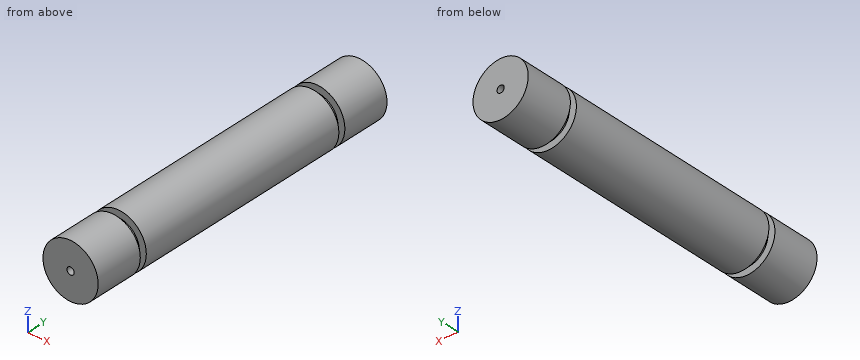
Autodesk Inventor part; units mm, degrees
ref_plane "YZ Plane" through (0, 0, 0) normal (1, 0, 0) x (0, 1, 0)
ref_plane "XZ Plane" through (0, 0, 0) normal (0, 1, 0) x (-1, 0, 0)
ref_plane "XY Plane" through (0, 0, 0) normal (0, 0, 1) x (1, 0, 0)
sketch "Sketch1" plane through (0, 0, 0) normal (0, 0, 1) x (1, 0, 0)
  line L0 (0, 0) -> (25.4, 0)
  line L1 (25.4, 304.8) -> (0, 304.8)
  line L2 (0, 304.8) -> (0, 0)
  line L3 (25.4, 44.45) -> (19.05, 44.45)
  line L4 (19.05, 44.45) -> (19.05, 50.8)
  line L5 (19.05, 50.8) -> (25.4, 50.8)
  line L6 (25.4, 254) -> (19.05, 254)
  line L7 (19.05, 254) -> (19.05, 260.35)
  line L8 (19.05, 260.35) -> (25.4, 260.35)
  line L9 (25.4, 260.35) -> (25.4, 304.8)
  line L10 (25.4, 0) -> (25.4, 44.45)
  line L11 (25.4, 50.8) -> (25.4, 254)
  point P0 (12.7, 152.4)
  point P1 (12.7, 0)
  dimension "d3" = 6.35
  dimension "d4" = 6.35
  dimension "d5" = 6.35
  dimension "d7" = 6.35
  dimension "d8" = 25.4
  dimension "d9" = 25.4
  dimension "d10" = 25.4
  dimension "d11" = 304.8
  dimension "d12" = 152.4
  dimension "d13" = 101.6
  dimension "d14" = 101.6
revolve "Revolution1" add sketch "Sketch1" angle 360 about axis through (0, 304.8, 0) along (0, -1, 0)
sketch "Sketch2" plane through (0, 304.8, 0) normal (0, 1, 0) x (1, 0, 0)
  point P0 (0, 0)
  point P1 (0, 0)
hole "Hole1" at (0, 304.8, 0) direction (0, -1, 0) diameter 6.604 end through all
properties part number "Roller" material "PVC-Piping"
Design review of the part built by this model. Coordinates are the model's own, in mm. Coordinates: 2 decimals unless noted, no trailing zeros. Write each loop counter-clockwise with the first axis right and the second up, starting at its lowest first coordinate (ties: lowest second). Pieces come first, ordered by that corner, then holes. Notation, with made-up numbers: (66, 9) -> (80, 9) arc R14 cw to (80, 13) -> close; hole circle Ø11 at (60.25, 73). An arc over 180 degrees is marked (long way). Write each question's results on one line, items separated by ' | '. Start each with the question number.
(1) Take a section at B-B on z = 0. Write out the cut boundary in (x, y).
(2) Take a section at D-D on z = 14. Write out the cut boundary in (x, y), and give its area (3 significant figures).
(3) For line 1 along Y through (x, z) = (-12, 16); line 2 along Z through (x, y) = (0, 126.5); line 3 along X through (y, z) = (263, -1), list the stretches that pass through material, from the lowest coordinate up. Write a range as from..to.
(4) Take a section at C-C on y = 163. Write out the cut boundary in (x, z).
(5) Take a section at A-A on x = 0. Write out the cut boundary in (y, z), and give its area (3 significant figures).
(6) Clearance check with flat-ended pins moving along their axes: P1, Ø4, axis at x = 3.5, y = 258, coming from the +Z side; P2, Ø12, axis at x = 15, y = 170.5, coming from the -Z side; P3, Ø15, axis at x = 7.5, z = 0, coming from the -Y side; P4, Ø1.5, axis at x = 4, y = 55.5, coming from the +Z side. State where each tip first meets the part, or that it passes through.
Results found:
1) outline: (-25.4, 0) -> (-3.3, 0) -> (-3.3, 304.8) -> (-25.4, 304.8) -> (-25.4, 260.35) -> (-19.05, 260.35) -> (-19.05, 254) -> (-25.4, 254) -> (-25.4, 50.8) -> (-19.05, 50.8) -> (-19.05, 44.45) -> (-25.4, 44.45) -> close; (3.3, 0) -> (25.4, 0) -> (25.4, 44.45) -> (19.05, 44.45) -> (19.05, 50.8) -> (25.4, 50.8) -> (25.4, 254) -> (19.05, 254) -> (19.05, 260.35) -> (25.4, 260.35) -> (25.4, 304.8) -> (3.3, 304.8) -> close
2) outline: (-21.19, 0) -> (21.19, 0) -> (21.19, 44.45) -> (12.92, 44.45) -> (12.92, 50.8) -> (21.19, 50.8) -> (21.19, 254) -> (12.92, 254) -> (12.92, 260.35) -> (21.19, 260.35) -> (21.19, 304.8) -> (-21.19, 304.8) -> (-21.19, 260.35) -> (-12.92, 260.35) -> (-12.92, 254) -> (-21.19, 254) -> (-21.19, 50.8) -> (-12.92, 50.8) -> (-12.92, 44.45) -> (-21.19, 44.45) -> close | area: 12,700 mm2
3) line 1: y = 0..44.45, 50.8..254, 260.35..304.8 | line 2: z = -25.4..-3.3, 3.3..25.4 | line 3: x = -25.38..-3.15, 3.15..25.38
4) outline: circle Ø50.8 at (0, 0); hole circle Ø6.6 at (0, 0)
5) outline: (0, -25.4) -> (44.45, -25.4) -> (44.45, -19.05) -> (50.8, -19.05) -> (50.8, -25.4) -> (254, -25.4) -> (254, -19.05) -> (260.35, -19.05) -> (260.35, -25.4) -> (304.8, -25.4) -> (304.8, -3.3) -> (0, -3.3) -> close; (0, 3.3) -> (304.8, 3.3) -> (304.8, 25.4) -> (260.35, 25.4) -> (260.35, 19.05) -> (254, 19.05) -> (254, 25.4) -> (50.8, 25.4) -> (50.8, 19.05) -> (44.45, 19.05) -> (44.45, 25.4) -> (0, 25.4) -> close | area: 13,300 mm2
6) P1: stops at z = 18.99 | P2: stops at z = -23.75 | P3: stops at y = 0 | P4: stops at z = 25.19
